```python
from build123d import *

# Parameters (mm, degrees)
SKETCH1_R           = 2.38125
SKETCH1_R_2         = 1.82245
BOSS_EXTRUDE1_DEPTH = 399.09877
SKETCH2_R           = 2.38125
BOSS_EXTRUDE2_DEPTH = 1.778
BOSS_EXTRUDE2_TAPER = -37
SKETCH3_R           = 1.82245
CUT_EXTRUDE1_DEPTH  = 2.7780001
CUT_EXTRUDE1_TAPER  = -37


with BuildPart() as part:
    # Sketch1 → Boss-Extrude1 (new body, symmetric)
    with BuildSketch(Plane.XY):
        Circle(SKETCH1_R)
        Circle(SKETCH1_R_2, mode=Mode.SUBTRACT)
    extrude(amount=BOSS_EXTRUDE1_DEPTH, both=True)

    # Sketch2 → Boss-Extrude2 (add)
    with BuildSketch(Plane.XY.offset(399.09877)):
        Circle(SKETCH2_R)
    boss_extrude2 = extrude(amount=BOSS_EXTRUDE2_DEPTH, taper=BOSS_EXTRUDE2_TAPER)

    # Sketch3 → Cut-Extrude1 (cut, through all)
    with BuildSketch(Plane(origin=(0, 0, 399.09877), x_dir=(-1, 0, 0), z_dir=(0, 0, -1))):
        Circle(SKETCH3_R)
    cut_extrude1 = extrude(amount=-CUT_EXTRUDE1_DEPTH, taper=CUT_EXTRUDE1_TAPER, mode=Mode.SUBTRACT)

    # Mirror1: Boss-Extrude2, Cut-Extrude1 across plane
    add(boss_extrude2.mirror(Plane.XY))
    add(cut_extrude1.mirror(Plane.XY), mode=Mode.SUBTRACT)


solid = part.part
```
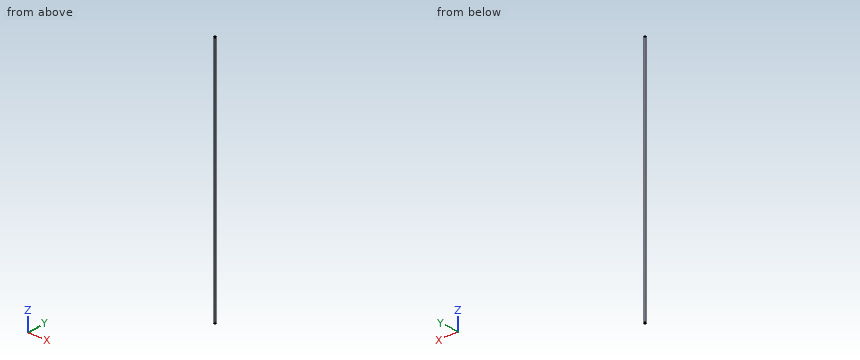
Input: part model. Units: mm. Frame: model coordinates. Coordinates: 2 decimals unless noted, no trailing zeros. Loops run counter-clockwise (first coordinate to the right, second up) from the corner with the lowest first, then second, coordinate; pieces in that order, holes last. Notation, with made-up numbers: M -19.5,48 L 4.5,48 A21 cw 4.5,57 Z; hole C -26,33 d11. An arc over 180 degrees is marked long. Use a Markdown table: item, result. Add a question column.
1) Pin query (flat end, axial travel): P1, Ø1.5, axis at x = -0.5, y = -1, coming from the -Z side; P2, Ø3, axis at x = -1.5, y = -0.5, coming from the +Z side; P3, Ø4, axis at x = -1.5, z = 103, coming from the +Y side. Return the tip coordinate at first contact, or that it passes through.
2) Section A-A, the plane x = 0. Return the cut outline in (y, z).
3) Section B-B, the plane z = -52. Return the cut outline in (x, y), plus the area to 3 significant figures.
4) Line query: L1, parallel to Y at x = 0, z = 213; L2, parallel to Z at x = 2, y = -3; L3, parallel to X at y = 0.5, z = -74. Output: solid intervals per line, ascending. Write a range as from..to.
Answer below:
| question | item | result |
|---|---|---|
| 1 | P1 | z = -399.16 |
| 1 | P2 | z = 400.77 |
| 1 | P3 | y = 2.38 |
| 2 | outline | M -3.72,-400.88 L -3.16,-400.88 L -1.82,-399.1 L -1.82,399.1 L -3.16,400.88 L -3.72,400.88 L -2.38,399.1 L -2.38,-399.1 Z; M 1.82,-399.1 L 3.16,-400.88 L 3.72,-400.88 L 2.38,-399.1 L 2.38,399.1 L 3.72,400.88 L 3.16,400.88 L 1.82,399.1 Z |
| 3 | outline | C 0,0 d4.76; hole C 0,0 d3.64 |
| 3 | area | 7.38 mm2 |
| 4 | L1 | -2.38..-1.82, 1.82..2.38 |
| 4 | L2 | -400.88..-400.72, 400.72..400.88 |
| 4 | L3 | -2.33..-1.75, 1.75..2.33 |
